```python
from build123d import *

# Parameters (mm, degrees)
SKETCH1_W           = 65
SKETCH1_H           = 50
BOSS_EXTRUDE1_DEPTH = 12
CUT_EXTRUDE1_DEPTH  = 6
SKETCH3_R           = 9
CUT_EXTRUDE2_DEPTH  = 7
SKETCH4_R           = 20.25
CUT_EXTRUDE3_DEPTH  = 3
SKETCH5_W           = 12
SKETCH5_H           = 50
BOSS_EXTRUDE2_DEPTH = 13
SKETCH6_W           = 8.2
SKETCH6_H           = 50
CUT_EXTRUDE4_DEPTH  = 5.7
SKETCH7_W           = 5
SKETCH7_H           = 50
BOSS_EXTRUDE3_DEPTH = 5
SKETCH8_W           = 5
SKETCH8_H           = 50
BOSS_EXTRUDE4_DEPTH = 5
FILLET1_R           = 2
FILLET2_R           = 2
BOSS_EXTRUDE6_DEPTH = 25
FILLET3_R           = 2
FILLET4_R           = 2
SKETCH10_W          = 1
SKETCH10_H          = 50
CUT_EXTRUDE5_DEPTH  = 7
SKETCH11_W          = 88
SKETCH11_H          = 1
CUT_EXTRUDE6_DEPTH  = 13
FILLET5_R           = 3
FILLET6_R           = 3
FILLET7_R           = 3
FILLET8_R           = 3


with BuildPart() as part:
    # Sketch1 → Boss-Extrude1 (new body)
    with BuildSketch(Plane.XY):
        Rectangle(SKETCH1_W, SKETCH1_H)
    extrude(amount=BOSS_EXTRUDE1_DEPTH)

    # Sketch2 → Cut-Extrude1 (cut)
    with BuildSketch(Plane.XY.offset(12)):
        with BuildLine():
            Line((-0.079165483, -16.163398081), (-1.679165483, -18.934679373))
            ThreePointArc((-1.679165483, -18.934679373), (15.625, -17.537014427), (25.487496091, -3.25))
            Line((25.487496091, -3.25), (22.287496091, -3.25))
            Line((22.287496091, -3.25), (22.287496091, 3.25))
            Line((22.287496091, 3.25), (25.487496091, 3.25))
            ThreePointArc((25.487496091, 3.25), (15.625, 17.537014427), (-1.679165483, 18.934679373))
            Line((-1.679165483, 18.934679373), (-0.079165483, 16.163398081))
            Line((-0.079165483, 16.163398081), (-5.708330608, 12.913398081))
            Line((-5.708330608, 12.913398081), (-7.308330608, 15.684679373))
            ThreePointArc((-7.308330608, 15.684679373), (-11.475017308, 11.041344456), (-14.030488985, 5.35))
            Line((-14.030488985, 5.35), (-14.030488985, -5.35))
            ThreePointArc((-14.030488985, -5.35), (-11.475017308, -11.041344456), (-7.308330608, -15.684679373))
            Line((-7.308330608, -15.684679373), (-5.708330608, -12.913398081))
            Line((-5.708330608, -12.913398081), (-0.079165483, -16.163398081))
        make_face()
        with BuildLine():
            Line((-44.030488985, -5.35), (-14.030488985, -5.35))
            ThreePointArc((-14.030488985, -5.35), (-14.75, 0), (-14.030488985, 5.35))
            Line((-14.030488985, 5.35), (-44.030488985, 5.35))
            Line((-44.030488985, 5.35), (-44.030488985, -5.35))
        make_face()
        with BuildLine():
            ThreePointArc((-14.030488985, 5.35), (-14.75, 0), (-14.030488985, -5.35))
            Line((-14.030488985, -5.35), (-14.030488985, 5.35))
        make_face()
    extrude(amount=-CUT_EXTRUDE1_DEPTH, mode=Mode.SUBTRACT)

    # Sketch3 → Cut-Extrude2 (cut, through all)
    with BuildSketch(Plane.XY.offset(6)):
        with Locations((5.5, 0)):
            Circle(SKETCH3_R)
    extrude(amount=-CUT_EXTRUDE2_DEPTH, mode=Mode.SUBTRACT)

    # Sketch4 → Cut-Extrude3 (cut)
    with BuildSketch(Plane.XY.offset(12)):
        with Locations((5.5, 0)):
            Circle(SKETCH4_R)
    extrude(amount=-CUT_EXTRUDE3_DEPTH, mode=Mode.SUBTRACT)

    # Sketch5 → Boss-Extrude2 (add)
    with BuildSketch(Plane(origin=(32.5, 0, 0), x_dir=(0, 0, -1), z_dir=(1, 0, 0))):
        with Locations((-6, 0)):
            Rectangle(SKETCH5_W, SKETCH5_H)
    extrude(amount=BOSS_EXTRUDE2_DEPTH)

    # Sketch6 → Cut-Extrude4 (cut)
    with BuildSketch(Plane.XY.offset(12)):
        with Locations((36.409019421, 0)):
            Rectangle(SKETCH6_W, SKETCH6_H)
    extrude(amount=-CUT_EXTRUDE4_DEPTH, mode=Mode.SUBTRACT)

    # Sketch7 → Boss-Extrude3 (add)
    with BuildSketch(Plane(origin=(45.5, 0, 0), x_dir=(0, 0, -1), z_dir=(1, 0, 0))):
        with Locations((-2.5, 0)):
            Rectangle(SKETCH7_W, SKETCH7_H)
    extrude(amount=BOSS_EXTRUDE3_DEPTH)

    # Sketch8 → Boss-Extrude4 (add)
    with BuildSketch(Plane.ZY.offset(32.5)):
        with Locations((2.5, 0)):
            Rectangle(SKETCH8_W, SKETCH8_H)
    extrude(amount=BOSS_EXTRUDE4_DEPTH)

    # Fillet1
    fillet1_edges = [part.edges().sort_by_distance(p)[0] for p in [
        (50.5, 0, 5),
    ]]
    fillet(fillet1_edges, radius=FILLET1_R)

    # Fillet2
    fillet2_edges = [part.edges().sort_by_distance(p)[0] for p in [
        (-37.5, 0, 5),
    ]]
    fillet(fillet2_edges, radius=FILLET2_R)

    # Sketch9 → Boss-Extrude6 (add)
    with BuildSketch(Plane.XY.offset(12)):
        with BuildLine():
            Line((-16.092960793, 10.475879161), (-12.705503837, 8.889726094))
            ThreePointArc((-12.705503837, 8.889726094), (10.062022154, 19.739694878), (25.76, 0))
            ThreePointArc((25.76, 0), (9.783964079, -19.801900206), (-12.948317056, -8.374198339))
            Line((-12.948317056, -8.374198339), (-16.391781636, -9.83615254))
            ThreePointArc((-16.391781636, -9.83615254), (10.529773391, -23.467027499), (29.5, 0))
            ThreePointArc((29.5, 0), (10.874427457, 23.390500839), (-16.092960793, 10.475879161))
        make_face()
    extrude(amount=BOSS_EXTRUDE6_DEPTH)

    # Fillet3
    fillet3_edges = [part.edges().sort_by_distance(p)[0] for p in [
        (-37.5, 0, 0),
    ]]
    fillet(fillet3_edges, radius=FILLET3_R)

    # Fillet4
    fillet4_edges = [part.edges().sort_by_distance(p)[0] for p in [
        (50.5, 0, 0),
    ]]
    fillet(fillet4_edges, radius=FILLET4_R)

    # Sketch10 → Cut-Extrude5 (cut)
    with BuildSketch(Plane.XY.offset(12)):
        with Locations((45, 0)):
            Rectangle(SKETCH10_W, SKETCH10_H)
        with Locations((-32, 0)):
            Rectangle(SKETCH10_W, SKETCH10_H)
    extrude(amount=-CUT_EXTRUDE5_DEPTH, mode=Mode.SUBTRACT)

    # Sketch11 → Cut-Extrude6 (cut, through all)
    with BuildSketch(Plane.XY.offset(12)):
        with Locations((6.5, -24.5)):
            Rectangle(SKETCH11_W, SKETCH11_H)
    extrude(amount=-CUT_EXTRUDE6_DEPTH, mode=Mode.SUBTRACT)

    # Fillet5
    fillet5_edges = [part.edges().sort_by_distance(p)[0] for p in [
        (44.5, -24, 8.5),
    ]]
    fillet(fillet5_edges, radius=FILLET5_R)

    # Fillet6
    fillet6_edges = [part.edges().sort_by_distance(p)[0] for p in [
        (44.5, 25, 8.5),
    ]]
    fillet(fillet6_edges, radius=FILLET6_R)

    # Fillet7
    fillet7_edges = [part.edges().sort_by_distance(p)[0] for p in [
        (-31.5, 25, 8.5),
    ]]
    fillet(fillet7_edges, radius=FILLET7_R)

    # Fillet8
    fillet8_edges = [part.edges().sort_by_distance(p)[0] for p in [
        (-31.5, -24, 8.5),
    ]]
    fillet(fillet8_edges, radius=FILLET8_R)


solid = part.part
```
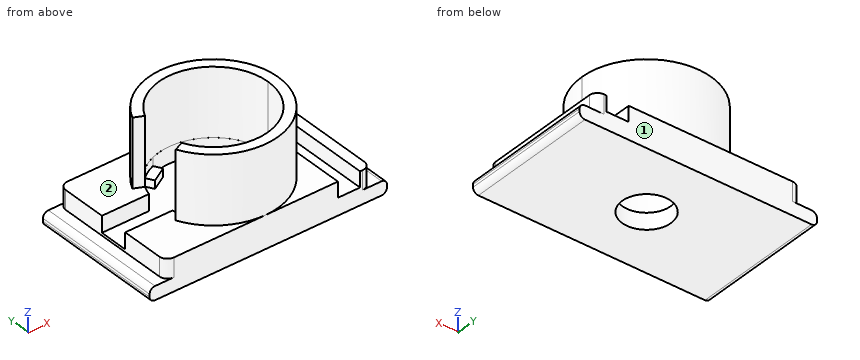
Design review of the part built by this model. Coordinates are the model's own, in mm. Face numbers are marked on the shaded views. A direction names the side the tool comes from. Coordinates: 2 decimals unless noted, no trailing zeros. Order: outer loops, then holes, each group sorted by start corner. A loop starts at its lowest first (then second) coordinate and runs counter-clockwise, first axis right, second up. Notation, with made-up numbers: (53.25, 26.25) -> (58.25, 26.25) arc R21 cw to (58.25, 44.25) -> close; hole circle Ø6 at (-20.5, 24). An arc over 180 degrees is marked (long way). One line per item, written item: value. Start each with the question number.
Q1. Take a section at D-D, the plane x = -20. State the section outline as (y, z) points.
Q2. For probe 1 along Y at (x, z) = (5.5, 3.6); probe 2 along Z at (x, y) = (-12.5, 6.5); probe 3 along X at (y, z) = (-9, 14), list the stretches that pass through material, from the lowest coordinate up.
Q3. Insertion check: pin 1 Ø1 at (y, z) = (-4.5, 14.5) entering from -X; pin 2 Ø11 at (x, y) = (5.5, 0) entering from -Z; pin 3 Ø7.5 at (x, y) = (-31, -11.5) entering from +Z; pin 4 Ø1 at (x, z) = (12.5, 27.5) entering from -Y. Each pin has a flat end and moves straight along its axis. Give the tip position at first contact, or say it passes through.
Q4. Tool access review of the marked faces 1 and 2: name each direction out of +Z, -Z, +X, -X, +Y, -Y from which nothing blocks a thin tool from reaching the whole face with its end or side.
Q5. Take a section at B-B, the plane z = 19.5. State the section outline as (x, y) points.
Values follow:
1. outline: (-24, 0) -> (25, 0) -> (25, 12) -> (5.35, 12) -> (5.35, 6) -> (-5.35, 6) -> (-5.35, 12) -> (-24, 12) -> close
2. probe 1: y = -24 to -9, 9 to 25
2. probe 2: z = 0 to 6
2. probe 3: x = -14.42 to -12.65, 23.65 to 27.75
3. pin 1: stops at x = 25.13
3. pin 2: passes through
3. pin 3: stops at z = 12
3. pin 4: stops at y = -23.1
4. face 1: +Z, -Z, +X, -X, +Y
4. face 2: +Z
5. outline: (-16.39, -9.84) arc R24 ccw (long way) to (-16.09, 10.48) -> (-12.71, 8.89) arc R20.26 cw (long way) to (-12.95, -8.37) -> close
